CAD build for the part. Positions are in the model's coordinates, mm. A direction names the side the tool comes from. Coordinates: 2 decimals unless noted, no trailing zeros. Order: outer loops, then holes, each group sorted by start corner. A loop starts at its lowest first (then second) coordinate and runs counter-clockwise, first axis right, second up. Notation, with made-up numbers: (64, 45.25) - (95, 45.25) arc R30 cw to (95, 76.25) - close; hole circle Ø6 at (44.25, 56.5). An arc over 180 degrees is marked (long way). Use one line per item in the form item = value.
```python
from build123d import *

# Parameters (mm, degrees)
SKETCH1_R           = 38.1
SKETCH1_R_2         = 34.121686747
BOSS_EXTRUDE1_DEPTH = 838.2


with BuildPart() as part:
    # Sketch1 → Boss-Extrude1 (new body)
    with BuildSketch(Plane(origin=(0, 0, 0), x_dir=(1, 0, 0), z_dir=(0, 1, 0))):
        with Locations(Location((0, 0, 0), (0, 0, 270))):
            Circle(SKETCH1_R)
        with Locations(Location((0, 0, 0), (0, 0, 270))):
            Circle(SKETCH1_R_2, mode=Mode.SUBTRACT)
    extrude(amount=BOSS_EXTRUDE1_DEPTH)

    # Sketch2 → Revolve1 (revolve)
    with BuildSketch(Plane(origin=(0, 0, 0), x_dir=(0, 0, -1), z_dir=(1, 0, 0))):
        Polygon((-38.1, 788.271478615), (-45.313643111, 788.271478615), (-45.313643111, 838.2), (-97.234227, 914.4), (-90.020583889, 914.4), (-38.1, 838.2), align=None)
    revolve(axis=Axis((0, 838.2, 0), (0, -1, 0)))


solid = part.part
```
Item 1: Drill centre lines: line 1 (X direction, y = 395.5, z = 0); line 2 (X direction, y = 185, z = -15); line 3 (Z direction, x = -28.5, y = 592.5). Where is each one in solid material? Low to high. Write a range as [from, to].
Derived:
line_1 = [-38.1, -34.12], [34.12, 38.1]
line_2 = [-35.02, -30.65], [30.65, 35.02]
line_3 = [-25.29, -18.76], [18.76, 25.29]
Item 2: 3-axis set-ups, long thin cutter, end or side, ignore diameter. For faces 4 (the face through (-23.183, 388.618, -30.235)), 5 (the face through (86, 914.4, 28)): which of +Z, -Z, +X, -X, +Y, -Y reach the whole face in a straight line?
Derived:
face_4 = -Y
face_5 = +Z, -Z, +X, -X, +Y
Item 3: Cut at C-C, the plane y = 612. Write the cut outline in (x, z).
Derived:
outline = circle Ø76.2 at (0, 0); hole circle Ø68.24 at (0, 0)
Item 4: Cut at B-B, the plane x = 0. Write the cut outline in (y, z).
Derived:
outline = (0, -38.1) - (788.27, -38.1) - (788.27, -45.31) - (838.2, -45.31) - (914.4, -97.23) - (914.4, -90.02) - (838.2, -38.1) - (838.2, -34.12) - (0, -34.12) - close; (0, 34.12) - (838.2, 34.12) - (838.2, 38.1) - (914.4, 90.02) - (914.4, 97.23) - (838.2, 45.31) - (788.27, 45.31) - (788.27, 38.1) - (0, 38.1) - close
Item 5: Drop flat-ended pins along their axis: pin 1 (5 mm diameter, centred on x = -26.5, z = 32.5, fed in from +Y); pin 2 (12 mm diameter, centred on y = 602, z = 31.5, fed in from +X); pin 3 (2 mm diameter, centred on x = -1, y = 710, fed in from +Z). Give the stop position or say it passes through.
Derived:
pin_1 = 847.5
pin_2 = 28.31
pin_3 = 38.1
Item 6: Two-plate mould, pull along X, no slides. Class faces 1 (the face through (40.2, 813.59, 20.91)), 2 (the face through (-37, 788.271, 10)), 3 (the face through (-20, 838.2, -28)): +X half, -X half, draft (parallel to the pull), parting line (faces both ways), or undercut.
Derived:
face_1 = parting line
face_2 = draft
face_3 = undercut
Item 7: Cut at A-A, the plane z = 0. Write the cut outline in (x, y), plus the area to 3 significant figures.
Derived:
outline = (-97.23, 914.4) - (-45.31, 838.2) - (-45.31, 788.27) - (-38.1, 788.27) - (-38.1, 0) - (-34.12, 0) - (-34.12, 838.2) - (-38.1, 838.2) - (-90.02, 914.4) - close; (34.12, 0) - (38.1, 0) - (38.1, 788.27) - (45.31, 788.27) - (45.31, 838.2) - (97.23, 914.4) - (90.02, 914.4) - (38.1, 838.2) - (34.12, 838.2) - close
area = 8,490 mm²
